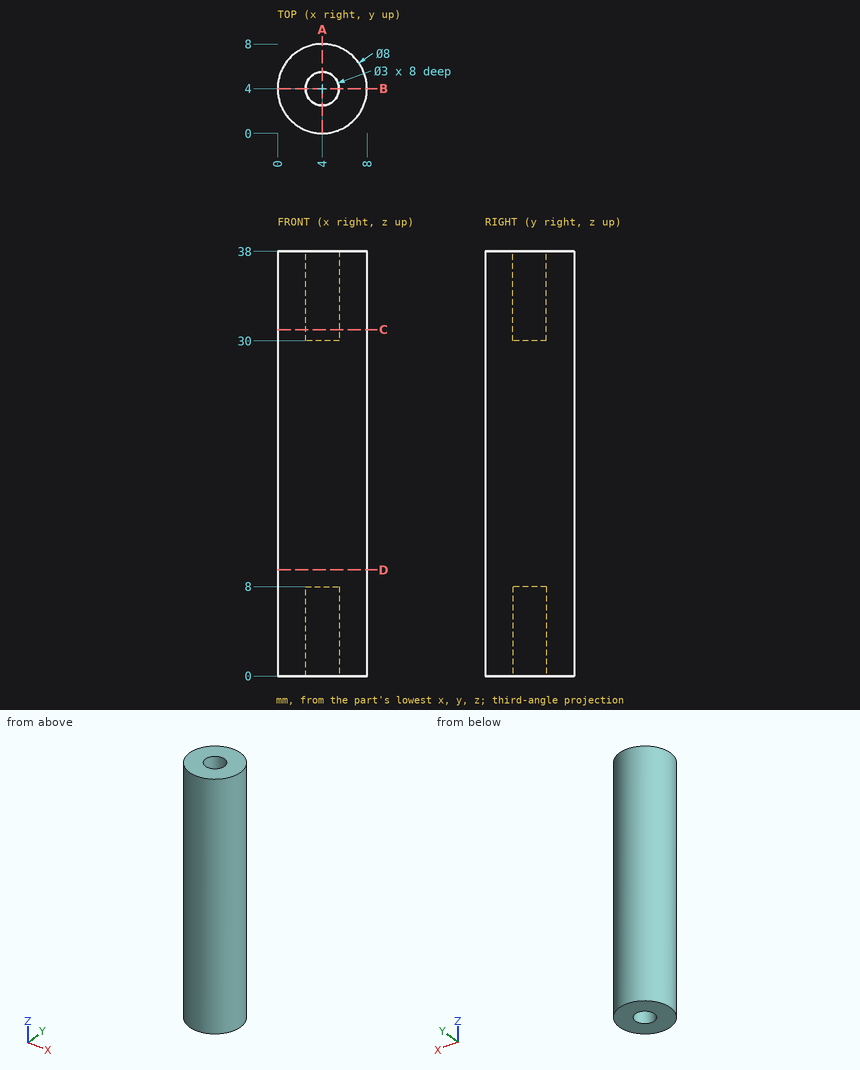
Part print with two shaded views. Sizes in mm from the minimum x, y, z corner. Round coordinates to 2 decimals unless told otherwise and drop trailing zeros. Order: outer loops, then holes, each group sorted by start corner. A loop starts at its lowest first (then second) coordinate and runs counter-clockwise, first axis right, second up. Notation, with made-up numbers: M -37,77.25 L -20,77.25 A18 ccw -20,102.25 Z; hole C -14.75,-8 d11. An arc over 180 degrees is marked long. Answer in a Markdown table with one row per item. Add a question column.
Q1. Cut at D-D on z = 9.5. Give the cut face in (x, y), and give its area (3 significant figures).
Q2. Wall check: L1, parallel to Y at x = 4, z = 2; L2, parallel to X at y = 4.25, z = 30.5; L3, parallel to Y at x = 2.75, z = 36.5. Give the ranges that are in metal, low to high. Write a range as from..to.
Q3. Cut at C-C on z = 31. Give the cut face in (x, y), and give its area (3 significant figures).
Q4. Cut at A-A on x = 4. Give the cut face in (y, z), and give its area (3 significant figures).
Q5. Pin check, flat tips, straight feed: pin 1 (1 mm diameter, centred on y = 2, z = 13, fed in from +X); pin 2 (2 mm diameter, centred on x = 6, z = 26, fed in from -Y); pin 3 (0.9 mm diameter, centred on x = 4.5, y = 4.5, fed in from +Z). Stop position of each tip, or through.
Established:
| question | item | result |
|---|---|---|
| 1 | outline | C 4,4 d8 |
| 1 | area | 50.3 mm2 |
| 2 | L1 | y = 0..2.5, 5.5..8 |
| 2 | L2 | x = 0.01..2.52, 5.48..7.99 |
| 2 | L3 | y = 0.2..3.17, 4.83..7.8 |
| 3 | outline | C 4,4 d8; hole C 4,4 d3 |
| 3 | area | 43.2 mm2 |
| 4 | outline | M 0,0 L 2.5,0 L 2.5,8 L 5.5,8 L 5.5,0 L 8,0 L 8,38 L 5.5,38 L 5.5,30 L 2.5,30 L 2.5,38 L 0,38 Z |
| 4 | area | 256 mm2 |
| 5 | pin 1 | stops at x = 7.71 |
| 5 | pin 2 | stops at y = 0.13 |
| 5 | pin 3 | stops at z = 30 |
